from build123d import *

# Parameters (mm, degrees)
F1_DEPTH = 2.54
F2_R     = 5.08
F3_R     = 10.16


with BuildPart() as f1:
    # F0 (on Front) → F1 (new body, symmetric)
    with BuildSketch(Plane.XZ):
        Polygon((-27.94, 0), (-22.86, 0), (-22.86, 10.16), (-2.54, 10.16), (-2.54, 0), (2.54, 0), (2.54, 10.16), (22.86, 10.16), (22.86, 0), (27.94, 0), (27.94, 15.24), (2.54, 15.24), (2.54, 25.4), (-2.54, 25.4), (-2.54, 15.24), (-27.94, 15.24), align=None)
    extrude(amount=F1_DEPTH, both=True)

    # F2
    f2_edges = [f1.edges().sort_by_distance(p)[0] for p in [
        (2.54, 0, 15.24),
        (2.54, 0, 10.16),
        (-2.54, 0, 10.16),
        (-2.54, 0, 15.24),
        (22.86, 0, 10.16),
        (-22.86, 0, 10.16),
    ]]
    fillet(f2_edges, radius=F2_R)

    # F3
    f3_edges = [f1.edges().sort_by_distance(p)[0] for p in [
        (27.94, 0, 15.24),
        (-27.94, 0, 15.24),
    ]]
    fillet(f3_edges, radius=F3_R)


solid = f1.part
Part model, mm, in its own coordinate system. A direction names the side the tool comes from. Coordinates: 2 decimals unless noted, no trailing zeros. Write each loop counter-clockwise with the first axis right and the second up, starting at its lowest first coordinate (ties: lowest second). Pieces come first, ordered by that corner, then holes. Notation, with made-up numbers: M 26.5,-8 L 44.5,-8 A17 cw 44.5,10 Z; hole C 79,62 d10. An arc over 180 degrees is marked long. Return JSON: item names as keys, results as strings.
1. Saw through at C-C, the plane x = -15. Write the cut outline in (y, z).
Determined:
{"outline": "M -2.54,10.16 L 2.54,10.16 L 2.54,15.24 L -2.54,15.24 Z"}
2. 3-axis set-ups, long thin cutter, end or side, ignore diameter. For faces 1 (the face through (2.54, 0, 23)), 2 (the face through (25, 0, 0)), 3 (the face through (-3.989, -0.036, 8.632)): which of +Z, -Z, +X, -X, +Y, -Y reach the whole face in a straight line?
Determined:
{"face 1": "+Z, +X, +Y, -Y", "face 2": "-Z, +X, -X, +Y, -Y", "face 3": "-Z, +Y, -Y"}
3. Flat gauge pins, fed straight in: pin 1 Ø1.5 at (y, z) = (-1, 22) entering from +X; pin 2 Ø2.5 at (x, y) = (-13.5, -0.5) entering from -Z; pin 3 Ø3 at (x, y) = (11.5, 0.5) entering from +Z. Where does each tip first touch, or does it go through?
Determined:
{"pin 1": "x = 2.54", "pin 2": "z = 10.16", "pin 3": "z = 15.24"}
4. Probe L1, parallel to X at y = -1.35, z = 3.75; L2, parallel to X at y = -1.6, z = 7.25; L3, parallel to X at y = -1.95, z = 21.75. List the from-to ranges inside material, lowest first.
Determined:
{"L1": "-27.94 to -22.86, -2.54 to 2.54, 22.86 to 27.94", "L2": "-27.71 to -22.37, -3.03 to 3.03, 22.37 to 27.71", "L3": "-2.54 to 2.54"}
5. Saw through at B-B, the plane y = 0.7. Write the cut outline in (x, z), then the cut area to 3 significant figures.
Determined:
{"outline": "M -27.94,0 L -22.86,0 L -22.86,5.08 A5.08 cw -17.78,10.16 L -7.62,10.16 A5.08 cw -2.54,5.08 L -2.54,0 L 2.54,0 L 2.54,5.08 A5.08 cw 7.62,10.16 L 17.78,10.16 A5.08 cw 22.86,5.08 L 22.86,0 L 27.94,0 L 27.94,5.08 A10.16 ccw 17.78,15.24 L 7.62,15.24 A5.08 cw 2.54,20.32 L 2.54,25.4 L -2.54,25.4 L -2.54,20.32 A5.08 cw -7.62,15.24 L -17.78,15.24 A10.16 ccw -27.94,5.08 Z", "area": "479 mm²"}
6. Saw through at A-A, the plane z = 4.5. Write the cut outline in (x, y), then the cut area to 3 significant figures.
Determined:
{"outline": "M -27.94,-2.54 L -22.86,-2.54 L -22.86,2.54 L -27.94,2.54 Z; M -2.54,-2.54 L 2.54,-2.54 L 2.54,2.54 L -2.54,2.54 Z; M 22.86,-2.54 L 27.94,-2.54 L 27.94,2.54 L 22.86,2.54 Z", "area": "77.4 mm²"}
7. Saw through at D-D, the plane z = 8. Write the cut outline in (x, y), then the cut area to 3 significant figures.
Determined:
{"outline": "M -27.51,-2.54 L -21.94,-2.54 L -21.94,2.54 L -27.51,2.54 Z; M -3.46,-2.54 L 3.46,-2.54 L 3.46,2.54 L -3.46,2.54 Z; M 21.94,-2.54 L 27.51,-2.54 L 27.51,2.54 L 21.94,2.54 Z", "area": "91.8 mm²"}
8. Pull direction X, two halves, no side cores. Call faces 4 (the face through (2.54, 0, 3)), 5 (the face through (0, -2.54, 11)), 6 (the face through (-4.068, 0.036, 16.689)), 7 (the face through (-21.332, -0.036, 8.711)): pulls with the +X half, pulls with the -X half, needs draft (parallel to the pull), parting line crosses it, or undercut.
Determined:
{"face 4": "undercut", "face 5": "needs draft", "face 6": "pulls with the -X half", "face 7": "undercut"}
